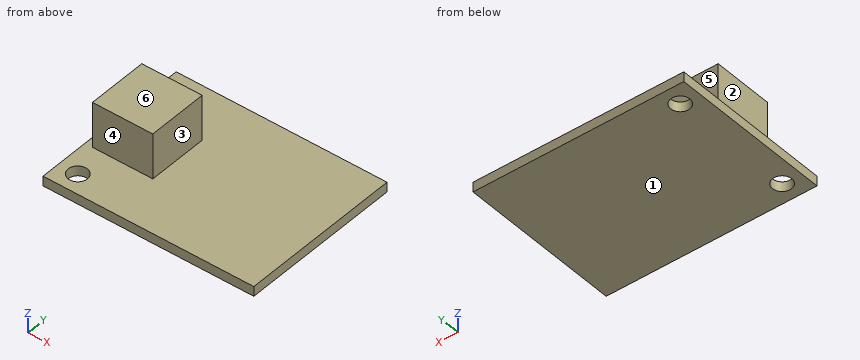
```python
from build123d import *

# Parameters (mm, degrees)
F0_W     = 27.94
F0_H     = 21.59
F0_R     = 1.27
F1_DEPTH = 0.65
F2_W     = 8
F2_H     = 8
F3_DEPTH = 6


with BuildPart() as f1:
    # F0 (on Top) → F1 (new body, symmetric)
    with BuildSketch(Plane.XY):
        Rectangle(F0_W, F0_H)
        with Locations((-11.43, -8.255)):
            Circle(F0_R, mode=Mode.SUBTRACT)
        with Locations((-11.43, 8.255)):
            Circle(F0_R, mode=Mode.SUBTRACT)
    extrude(amount=F1_DEPTH, both=True)

    # F2 (on face) → F3 (join)
    with BuildSketch(Plane.XY.offset(0.65)):
        with Locations((-8.97, 0)):
            Rectangle(F2_W, F2_H)
    extrude(amount=F3_DEPTH)


solid = f1.part
```
Geometry check sheet. Reference: the model listing, model coordinates, mm. Face numbers are marked on the shaded views. A direction names the side the tool comes from. Coordinates: 2 decimals unless noted, no trailing zeros. Loops run counter-clockwise (first coordinate to the right, second up) from the corner with the lowest first, then second, coordinate; pieces in that order, holes last. Notation, with made-up numbers: (56, -40) - (107, -40) arc R21 cw to (107, -24) - close; hole circle Ø11 at (47.25, 86.25). An arc over 180 degrees is marked (long way). One line per item, written item: value. Start each with the question number.
(1) Tool access check on the marked faces 4, 5 and 6. Record the directions out of +Z, -Z, +X, -X, +Y, -Y that give a thin tool (end or side, any length) a straight path to the whole face; none if there is none.
(2) Cross-section at C-C on y = -1.5. Enter the section's corners in (x, z), plus the area to 3 significant figures.
(3) Cross-section at D-D on x = 0.5. Enter the section's corners in (y, z) (3 decimals).
(4) Mould release check, pull along X, two halves, no side actions. Record for the marked faces 1, 2 and 3: released by +X, released by -X, zero draft, split by the parting line, or undercut.
(5) Cross-section at A-A on x = -11.43. Enter the section's corners in (y, z) (3 decimals), plus the area to 3 significant figures.
(6) Material ranges on line 1 (Y direction, x = -11.43, z = 0.35) (3 decimals); line 2 (Z direction, x = 12.5, y = 8.5); line 3 (X direction, y = 2.25, z = 2), recorded low to high. Write a range as [from, to].
(7) Cross-section at B-B on y = 7.5. Enter the section's corners in (x, z), plus the area to 3 significant figures.
(8) Depth check by flat-ended pin: P1, Ø1.5, axis at x = -7.5, z = 4.5, coming from the +Y side; P2, Ø1.8, axis at y = -0.5, z = 5, coming from the -X side; P3, Ø3, axis at x = -8, z = 2.5, coming from the -Y side; P4, Ø3.5, axis at x = -11.43, y = 8.255, coming from the -Z side. Enter the tip coordinate at first touch or a pass-through.
Results below:
1. face 4: +Z, +X, -X, -Y
1. face 5: +Z, +X, -X, +Y
1. face 6: +Z, +X, -X, +Y, -Y
2. outline: (-13.97, -0.65) - (13.97, -0.65) - (13.97, 0.65) - (-4.97, 0.65) - (-4.97, 6.65) - (-12.97, 6.65) - (-12.97, 0.65) - (-13.97, 0.65) - close
2. area: 84.3 mm2
3. outline: (-10.795, -0.65) - (10.795, -0.65) - (10.795, 0.65) - (-10.795, 0.65) - close
4. face 1: zero draft
4. face 2: released by -X
4. face 3: released by +X
5. outline: (-10.795, -0.65) - (-9.525, -0.65) - (-9.525, 0.65) - (-10.795, 0.65) - close; (-6.985, -0.65) - (6.985, -0.65) - (6.985, 0.65) - (4, 0.65) - (4, 6.65) - (-4, 6.65) - (-4, 0.65) - (-6.985, 0.65) - close; (9.525, -0.65) - (10.795, -0.65) - (10.795, 0.65) - (9.525, 0.65) - close
5. area: 69.5 mm2
6. line 1: y = [-10.795, -9.525], [-6.985, 6.985], [9.525, 10.795]
6. line 2: z = [-0.65, 0.65]
6. line 3: x = [-12.97, -4.97]
7. outline: (-13.97, -0.65) - (-12.45, -0.65) - (-12.45, 0.65) - (-13.97, 0.65) - close; (-10.41, -0.65) - (13.97, -0.65) - (13.97, 0.65) - (-10.41, 0.65) - close
7. area: 33.7 mm2
8. P1: stops at y = 4
8. P2: stops at x = -12.97
8. P3: stops at y = -4
8. P4: stops at z = -0.65
